from build123d import *

# Parameters (mm, degrees)
SKETCH1_W           = 20
SKETCH1_H           = 20
BOSS_EXTRUDE1_DEPTH = 3.5
SKETCH2_R           = 5
BOSS_EXTRUDE2_DEPTH = 10
CHAMFER1_SIZE       = 10
CHAMFER1_SIZE_2     = 1.763269807
FILLET1_R           = 5
FILLET2_R           = 5
SKETCH9_W           = 2
SKETCH9_H           = 8
BOSS_EXTRUDE4_DEPTH = 4
SKETCH10_W          = 7
SKETCH10_H          = 8
BOSS_EXTRUDE5_DEPTH = 1.5
FILLET3_SIZE        = 0.5
FILLET3_SIZE_2      = 1


# Read off the part's stored shape, not the designer's step: Revolve5
with BuildPart() as part:
    # Sketch1 → Boss-Extrude1 (new body)
    with BuildSketch(Plane(origin=(0, 0, 0), x_dir=(1, 0, 0), z_dir=(0, 1, 0))):
        Rectangle(SKETCH1_W, SKETCH1_H)
    extrude(amount=BOSS_EXTRUDE1_DEPTH)

    # Sketch2 → Boss-Extrude2 (add)
    with BuildSketch(Plane(origin=(0, 3.5, 0), x_dir=(1, 0, 0), z_dir=(0, 1, 0))):
        with Locations(Location((0, 0, 0), (0, 0, 270))):
            Circle(SKETCH2_R)
    extrude(amount=BOSS_EXTRUDE2_DEPTH)

    # Chamfer1
    # the kernel refuses this chamfer: 10, 1.763269807 mm, written as the material it takes off along each edge
    with BuildSketch(Plane(origin=(0, 13.5, 0), x_dir=(0, 0, 1), z_dir=(-1, 0, 0))) as chamfer1_piece_1_section:
        Polygon((5, -CHAMFER1_SIZE), (5 - CHAMFER1_SIZE_2, 0), (5, 0), align=None)
    chamfer1_piece_1 = revolve(axis=Axis((0, 13.5, 0), (0, 1, 0)), mode=Mode.PRIVATE)
    chamfer1_piece_1 = split(chamfer1_piece_1, bisect_by=Plane(origin=(0, 3.5, -4.151256053), z_dir=(0, 1, 0)), keep=Keep.TOP, mode=Mode.PRIVATE)
    add(chamfer1_piece_1, mode=Mode.SUBTRACT)

    # Fillet1
    fillet1_edges = [part.edges().sort_by_distance(p)[0] for p in [
        (10, 1.75, 10),
        (-10, 1.75, 10),
        (-10, 1.75, -10),
        (10, 1.75, -10),
    ]]
    fillet(fillet1_edges, radius=FILLET1_R)

    # Revolve5 outline → Revolve5 (revolve)
    with BuildSketch(Plane.XY):
        with BuildLine():
            ThreePointArc((3.320470439, 13.025085423), (7.303658649, 21.454866662), (0, 27.25))
            Line((0, 27.25), (0, 13.5))
            Line((0, 13.5), (3.236730193, 13.5))
            Line((3.236730193, 13.5), (3.236730193, 13.025085423))
            Line((3.236730193, 13.025085423), (3.320470439, 13.025085423))
        make_face()
    revolve(axis=Axis((0, 0, 0), (0, 1, 0)))

    # Fillet2
    fillet2_edges = [part.edges().sort_by_distance(p)[0] for p in [
        (0, 3.5, -5),
    ]]
    fillet(fillet2_edges, radius=FILLET2_R)

    # Sketch9 → Boss-Extrude4 (add)
    with BuildSketch(Plane.XZ):
        Rectangle(SKETCH9_W, SKETCH9_H)
    extrude(amount=BOSS_EXTRUDE4_DEPTH)

    # Sketch10 → Boss-Extrude5 (add)
    with BuildSketch(Plane(origin=(0, -4, 0), x_dir=(-1, 0, 0), z_dir=(0, -1, 0))):
        Rectangle(SKETCH10_W, SKETCH10_H)
    extrude(amount=BOSS_EXTRUDE5_DEPTH)

    # Fillet3
    # an asymmetric fillet: 1, 0.5 mm, written as the material it adds along each edge
    with BuildSketch(Plane(origin=(1, 0, -4), x_dir=(0, -1, 0), z_dir=(0, 0, 1)), Plane(origin=(-1, 0, 4), x_dir=(0, -1, 0), z_dir=(0, 0, -1))) as fillet3_piece_1:
        with BuildLine():
            Bezier((FILLET3_SIZE, 0), (0, 0), (0, FILLET3_SIZE_2), weights=[1, 0.707106781, 1])
            Line((0, FILLET3_SIZE_2), (0, 0))
            Line((0, 0), (FILLET3_SIZE, 0))
        make_face()
    extrude(amount=8)
    with BuildSketch(Plane(origin=(1, 0, 4), x_dir=(0, -1, 0), z_dir=(-1, 0, 0)), Plane(origin=(-1, 0, -4), x_dir=(0, -1, 0), z_dir=(1, 0, 0))) as fillet3_piece_2:
        with BuildLine():
            Bezier((FILLET3_SIZE, 0), (0, 0), (0, FILLET3_SIZE_2), weights=[1, 0.707106781, 1])
            Line((0, FILLET3_SIZE_2), (0, 0))
            Line((0, 0), (FILLET3_SIZE, 0))
        make_face()
    extrude(amount=2)
    with BuildSketch(Plane(origin=(-1, 0, -4), x_dir=(0, -1, 0), z_dir=(1, 0, 0))) as fillet3_piece_3a_section:
        with BuildLine():
            Bezier((FILLET3_SIZE, 0), (0, 0), (0, FILLET3_SIZE_2), weights=[1, 0.707106781, 1])
            Line((0, FILLET3_SIZE_2), (0, 0))
            Line((0, 0), (FILLET3_SIZE, 0))
        make_face()
    fillet3_piece_3a = extrude(amount=4.5, mode=Mode.PRIVATE)
    fillet3_piece_3a = split(fillet3_piece_3a, bisect_by=Plane(origin=(1, -0.103701438, -4.24592111), z_dir=(1, 0, 0)), keep=Keep.TOP, mode=Mode.PRIVATE)
    with BuildSketch(Plane(origin=(1, 0, -6.5), x_dir=(0, -1, 0), z_dir=(0, 0, 1))) as fillet3_piece_3b_section:
        with BuildLine():
            Bezier((FILLET3_SIZE, 0), (0, 0), (0, FILLET3_SIZE_2), weights=[1, 0.707106781, 1])
            Line((0, FILLET3_SIZE_2), (0, 0))
            Line((0, 0), (FILLET3_SIZE, 0))
        make_face()
    fillet3_piece_3b = extrude(amount=10.5, mode=Mode.PRIVATE)
    fillet3_piece_3b = split(fillet3_piece_3b, bisect_by=Plane(origin=(1.245921261, -0.103701518, -4), z_dir=(0, 0, -1)), keep=Keep.TOP, mode=Mode.PRIVATE)
    fillet3_piece_3 = fillet3_piece_3a & fillet3_piece_3b
    add(fillet3_piece_3)
    with BuildSketch(Plane(origin=(3.5, 0, 4), x_dir=(0, -1, 0), z_dir=(-1, 0, 0))) as fillet3_piece_4a_section:
        with BuildLine():
            Bezier((FILLET3_SIZE, 0), (0, 0), (0, FILLET3_SIZE_2), weights=[1, 0.707106781, 1])
            Line((0, FILLET3_SIZE_2), (0, 0))
            Line((0, 0), (FILLET3_SIZE, 0))
        make_face()
    fillet3_piece_4a = extrude(amount=4.5, mode=Mode.PRIVATE)
    fillet3_piece_4a = split(fillet3_piece_4a, bisect_by=Plane(origin=(1, -0.103701518, 4.245921261), z_dir=(1, 0, 0)), keep=Keep.TOP, mode=Mode.PRIVATE)
    with BuildSketch(Plane(origin=(1, 0, -4), x_dir=(0, -1, 0), z_dir=(0, 0, 1))) as fillet3_piece_4b_section:
        with BuildLine():
            Bezier((FILLET3_SIZE, 0), (0, 0), (0, FILLET3_SIZE_2), weights=[1, 0.707106781, 1])
            Line((0, FILLET3_SIZE_2), (0, 0))
            Line((0, 0), (FILLET3_SIZE, 0))
        make_face()
    fillet3_piece_4b = extrude(amount=10.5, mode=Mode.PRIVATE)
    fillet3_piece_4b = split(fillet3_piece_4b, bisect_by=Plane(origin=(1.24592111, -0.103701438, 4), z_dir=(0, 0, 1)), keep=Keep.TOP, mode=Mode.PRIVATE)
    fillet3_piece_4 = fillet3_piece_4a & fillet3_piece_4b
    add(fillet3_piece_4)
    with BuildSketch(Plane(origin=(1, 0, 4), x_dir=(0, -1, 0), z_dir=(-1, 0, 0))) as fillet3_piece_5a_section:
        with BuildLine():
            Bezier((FILLET3_SIZE, 0), (0, 0), (0, FILLET3_SIZE_2), weights=[1, 0.707106781, 1])
            Line((0, FILLET3_SIZE_2), (0, 0))
            Line((0, 0), (FILLET3_SIZE, 0))
        make_face()
    fillet3_piece_5a = extrude(amount=4.5, mode=Mode.PRIVATE)
    fillet3_piece_5a = split(fillet3_piece_5a, bisect_by=Plane(origin=(-1, -0.103701438, 4.24592111), z_dir=(-1, 0, 0)), keep=Keep.TOP, mode=Mode.PRIVATE)
    with BuildSketch(Plane(origin=(-1, 0, 6.5), x_dir=(0, -1, 0), z_dir=(0, 0, -1))) as fillet3_piece_5b_section:
        with BuildLine():
            Bezier((FILLET3_SIZE, 0), (0, 0), (0, FILLET3_SIZE_2), weights=[1, 0.707106781, 1])
            Line((0, FILLET3_SIZE_2), (0, 0))
            Line((0, 0), (FILLET3_SIZE, 0))
        make_face()
    fillet3_piece_5b = extrude(amount=10.5, mode=Mode.PRIVATE)
    fillet3_piece_5b = split(fillet3_piece_5b, bisect_by=Plane(origin=(-1.245921261, -0.103701518, 4), z_dir=(0, 0, 1)), keep=Keep.TOP, mode=Mode.PRIVATE)
    fillet3_piece_5 = fillet3_piece_5a & fillet3_piece_5b
    add(fillet3_piece_5)
    with BuildSketch(Plane(origin=(-3.5, 0, -4), x_dir=(0, -1, 0), z_dir=(1, 0, 0))) as fillet3_piece_6a_section:
        with BuildLine():
            Bezier((FILLET3_SIZE, 0), (0, 0), (0, FILLET3_SIZE_2), weights=[1, 0.707106781, 1])
            Line((0, FILLET3_SIZE_2), (0, 0))
            Line((0, 0), (FILLET3_SIZE, 0))
        make_face()
    fillet3_piece_6a = extrude(amount=4.5, mode=Mode.PRIVATE)
    fillet3_piece_6a = split(fillet3_piece_6a, bisect_by=Plane(origin=(-1, -0.103701518, -4.245921261), z_dir=(-1, 0, 0)), keep=Keep.TOP, mode=Mode.PRIVATE)
    with BuildSketch(Plane(origin=(-1, 0, 4), x_dir=(0, -1, 0), z_dir=(0, 0, -1))) as fillet3_piece_6b_section:
        with BuildLine():
            Bezier((FILLET3_SIZE, 0), (0, 0), (0, FILLET3_SIZE_2), weights=[1, 0.707106781, 1])
            Line((0, FILLET3_SIZE_2), (0, 0))
            Line((0, 0), (FILLET3_SIZE, 0))
        make_face()
    fillet3_piece_6b = extrude(amount=10.5, mode=Mode.PRIVATE)
    fillet3_piece_6b = split(fillet3_piece_6b, bisect_by=Plane(origin=(-1.24592111, -0.103701438, -4), z_dir=(0, 0, -1)), keep=Keep.TOP, mode=Mode.PRIVATE)
    fillet3_piece_6 = fillet3_piece_6a & fillet3_piece_6b
    add(fillet3_piece_6)


solid = part.part
Geometry: final body of the model. Coordinates: model frame, mm. A direction names the side the tool comes from. Give positions to 0.01 mm unless a question says otherwise; leave off trailing zeros. Order: outer loops, then holes, each group sorted by start corner. A loop starts at its lowest first (then second) coordinate and runs counter-clockwise, first axis right, second up. Notation, with made-up numbers: (80, -21) -> (111, -21) arc R21 ccw to (111, 13) -> close; hole circle Ø8 at (-31, 16). An arc over 180 degrees is marked (long way). Write each question's results on one line, items separated by ' | '.
1) Cut plane B-B (y = 16). Output: boundary loops of the cut face in (x, z), and give its area (3 significant figures).
Geometry says:
outline: circle Ø12.99 at (0, 0) | area: 133 mm²
2) First-contact query: pin 1 Ø1 at (x, y) = (4.5, 15.5) entering from +Z; pin 2 Ø0.8 at (y, z) = (-4.5, 0.5) entering from +X; pin 3 Ø12 at (y, z) = (16, 8) entering from -X. Flat tips, straight axial feed; report the tip coordinate or a pass-through.
Geometry says:
pin 1: stops at z = 4.89 | pin 2: stops at x = 3.5 | pin 3: stops at x = -6.94
3) Line query: line 1 along Y through (x, z) = (7.75, -6); line 2 along Y through (x, z) = (-4.5, -2.25); line 3 along Y through (x, z) = (6.5, -2.5). Output: solid intervals per line, ascending.
Geometry says:
line 1: y = 0 to 3.5 | line 2: y = 0 to 5.73, 14.19 to 25.31 | line 3: y = 0 to 4.03, 16.97 to 22.53
4) Draft query along Y for faces 5 (the face through (0, -5.5, 0)), 6 (the face through (3.5, -5, 0)), 7 (the face through (1.11, 10.97, 3.51)). Return one class per face: released by +Y, released by -Y, zero draft, split by the parting line, or undercut.
Geometry says:
face 5: released by -Y | face 6: zero draft | face 7: undercut
5) Set-up query: faces 1 (the face through (-1, -2, 0)), 2 (the face through (0, -4, -4)), 3 (the face through (-6, 3.5, -7.5)), 4 (the face through (2, -4, 0)). Return all of +Z, -Z, +X, -X, +Y, -Y with unobstructed straight access to the full face (end or side cutting, diameter ignored); none if empty.
Geometry says:
face 1: +Z, -Z, -X | face 2: -Z, +X, -X, -Y | face 3: +Y | face 4: +Z, -Z, +X
6) Cut plane A-A (y = 1). Output: boundary loops of the cut face in (x, z).
Geometry says:
outline: (-10, -5) arc R5 ccw to (-5, -10) -> (5, -10) arc R5 ccw to (10, -5) -> (10, 5) arc R5 ccw to (5, 10) -> (-5, 10) arc R5 ccw to (-10, 5) -> close
